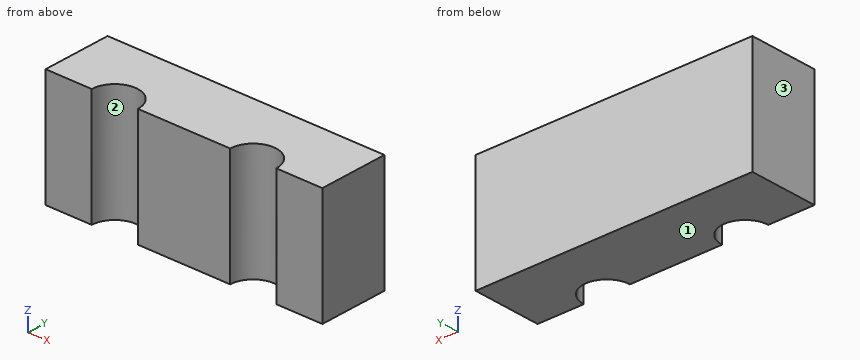
```python
from build123d import *

# Parameters (mm, degrees)
F1_DEPTH = 25


with BuildPart() as f1:
    # F0 (on Top) → F1 (new body)
    with BuildSketch(Plane.XY):
        with BuildLine():
            Line((-5.199284, -16.374299), (-65.199284, -16.374299))
            Line((-65.199284, -16.374299), (-65.199284, -31.374299))
            Line((-65.199284, -31.374299), (-55.199284, -31.374299))
            ThreePointArc((-55.199284, -31.374299), (-50.199284, -26.374299), (-45.199284, -31.374299))
            Line((-45.199284, -31.374299), (-25.199284, -31.374299))
            ThreePointArc((-25.199284, -31.374299), (-20.199284, -26.374299), (-15.199284, -31.374299))
            Line((-15.199284, -31.374299), (-5.199284, -31.374299))
            Line((-5.199284, -31.374299), (-5.199284, -16.374299))
        make_face()
    extrude(amount=F1_DEPTH)


solid = f1.part
```
Geometry: final body of the model. Coordinates: model frame, mm. Face numbers are marked on the shaded views. Coordinates: 2 decimals unless noted, no trailing zeros. Order: outer loops, then holes, each group sorted by start corner. A loop starts at its lowest first (then second) coordinate and runs counter-clockwise, first axis right, second up. Notation, with made-up numbers: (78.5, 32) -> (87.5, 32) arc R23 ccw to (87.5, 40) -> close; hole circle Ø9 at (30.25, -31). An arc over 180 degrees is marked (long way). Answer in a Markdown table with one row per item.
Item 1: Draft query along X for the marked faces 1, 2 and 3. Return one class per face: released by +X, released by -X, zero draft, split by the parting line, or undercut.
Return value:
| item | result |
|---|---|
| face 1 | zero draft |
| face 2 | undercut |
| face 3 | released by -X |
Item 2: Section B-B on y = -29.5. Output: boundary loops of the cut face in (x, z), plus the area to 3 significant figures.
Return value:
| item | result |
|---|---|
| outline | (-65.2, 0) -> (-54.83, 0) -> (-54.83, 25) -> (-65.2, 25) -> close; (-45.56, 0) -> (-24.83, 0) -> (-24.83, 25) -> (-45.56, 25) -> close; (-15.56, 0) -> (-5.2, 0) -> (-5.2, 25) -> (-15.56, 25) -> close |
| area | 1,040 mm² |
Item 3: Section D-D on x = -53. Output: boundary loops of the cut face in (y, z).
Return value:
| item | result |
|---|---|
| outline | (-27.23, 0) -> (-16.37, 0) -> (-16.37, 25) -> (-27.23, 25) -> close |
Item 4: Section C-C on x = -16. Output: boundary loops of the cut face in (y, z), plus the area to 3 significant figures.
Return value:
| item | result |
|---|---|
| outline | (-28.66, 0) -> (-16.37, 0) -> (-16.37, 25) -> (-28.66, 25) -> close |
| area | 307 mm² |
Item 5: Section A-A on z = 13.25. Output: boundary loops of the cut face in (x, y), plus the area to 3 significant figures.
Return value:
| item | result |
|---|---|
| outline | (-65.2, -31.37) -> (-55.2, -31.37) arc R5 cw to (-45.2, -31.37) -> (-25.2, -31.37) arc R5 cw to (-15.2, -31.37) -> (-5.2, -31.37) -> (-5.2, -16.37) -> (-65.2, -16.37) -> close |
| area | 821 mm² |
Item 6: Ray query, L1, parallel to X at y = -30.5, z = 8; L2, parallel to X at y = -29.5, z = 17.25; L3, parallel to Y at x = -47.5, z = 23.25. Return the intervals inside material, ascending.
Return value:
| item | result |
|---|---|
| L1 | x = -65.2 to -55.12, -45.28 to -25.12, -15.28 to -5.2 |
| L2 | x = -65.2 to -54.83, -45.56 to -24.83, -15.56 to -5.2 |
| L3 | y = -27.17 to -16.37 |
